from build123d import *

# Parameters (mm, degrees)
F1_DEPTH = 0.75
F2_W     = 0.8
F2_H     = 1
F3_DEPTH = 0.751
F4_W     = 0.8
F4_H     = 1
F5_DEPTH = 0.751
F6_W     = 0.8
F6_H     = 1
F7_DEPTH = 0.751
F8_W     = 0.8
F8_H     = 1
F9_DEPTH = 0.751


with BuildPart() as f1:
    # F0 (on Front) → F1 (new body)
    with BuildSketch(Plane.XZ):
        Polygon((11.8536589885, 0), (-20.1463410115, 0), (-20.1463410115, -3), (-8.1463410115, -3), (-8.1463410115, -1.2), (-0.1463410115, -1.2), (-0.1463410115, -3), (11.8536589885, -3), align=None)
    extrude(amount=F1_DEPTH)

    # F2 (on face) → F3 (cut, through all)
    with BuildSketch(Plane.XZ.offset(0.75)):
        with Locations((-19.2463410115, -0.5)):
            Rectangle(F2_W, F2_H)
    extrude(amount=-F3_DEPTH, mode=Mode.SUBTRACT)

    # F4 (on face) → F5 (cut, through all)
    with BuildSketch(Plane.XZ.offset(0.75)):
        with Locations((-8.5463410115, -0.5)):
            Rectangle(F4_W, F4_H)
    extrude(amount=-F5_DEPTH, mode=Mode.SUBTRACT)

    # F6 (on face) → F7 (cut, through all)
    with BuildSketch(Plane.XZ.offset(0.75)):
        with Locations((0.2536589885, -0.5)):
            Rectangle(F6_W, F6_H)
    extrude(amount=-F7_DEPTH, mode=Mode.SUBTRACT)

    # F8 (on face) → F9 (cut, through all)
    with BuildSketch(Plane.XZ.offset(0.75)):
        with Locations((10.9536589885, -0.5)):
            Rectangle(F8_W, F8_H)
    extrude(amount=-F9_DEPTH, mode=Mode.SUBTRACT)


solid = f1.part
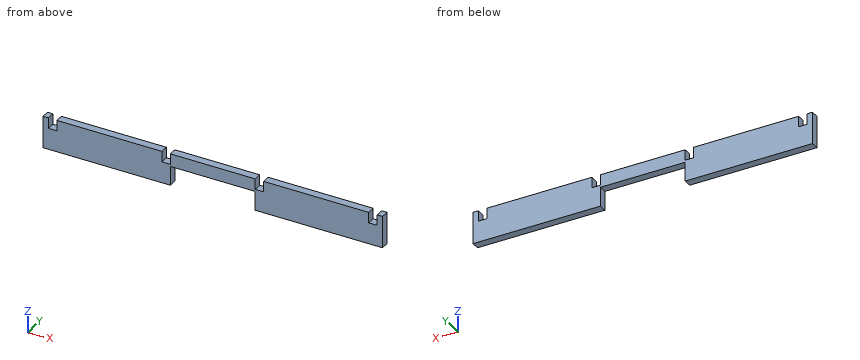
Check sheet for the modelled part. Datum: model origin and axes. Units: mm. Round coordinates to 2 decimals unless told otherwise and drop trailing zeros. Write each loop counter-clockwise with the first axis right and the second up, starting at its lowest first coordinate (ties: lowest second). Pieces come first, ordered by that corner, then holes. Notation, with made-up numbers: (31.25, -28.75) -> (90.25, -28.75) arc R30 ccw to (90.25, 0.25) -> close; hole circle Ø10 at (-7.5, -3.5). An arc over 180 degrees is marked (long way). Answer as CSV lines item,"result". Start each with the question number.
1) Section check A-A on z = -0.7. Enter the section's corners in (x, y).
2) Material ranges on line 1 (X direction, y = -0.05, z = -0.75); line 2 (X direction, y = -0.15, z = -1.35); line 3 (Z direction, x = -2, y = -0.35), recorded low to high. Write a range as from..to.
3) Section check D-D on x = -3.5. Enter the section's corners in (y, z).
4) Section check B-B on z = -2.45. Enter the section's corners in (x, y).
5) Section check C-C on y = -0.35. Enter the section's corners in (x, z).
Found:
1,outline,"(-20.15, -0.75) -> (-19.65, -0.75) -> (-19.65, 0) -> (-20.15, 0) -> close; (-18.85, -0.75) -> (-8.95, -0.75) -> (-8.95, 0) -> (-18.85, 0) -> close; (-8.15, -0.75) -> (-0.15, -0.75) -> (-0.15, 0) -> (-8.15, 0) -> close; (0.65, -0.75) -> (10.55, -0.75) -> (10.55, 0) -> (0.65, 0) -> close; (11.35, -0.75) -> (11.85, -0.75) -> (11.85, 0) -> (11.35, 0) -> close"
2,line 1,"x = -20.15..-19.65, -18.85..-8.95, -8.15..-0.15, 0.65..10.55, 11.35..11.85"
2,line 2,"x = -20.15..-8.15, -0.15..11.85"
2,line 3,"z = -1.2..0"
3,outline,"(-0.75, -1.2) -> (0, -1.2) -> (0, 0) -> (-0.75, 0) -> close"
4,outline,"(-20.15, -0.75) -> (-8.15, -0.75) -> (-8.15, 0) -> (-20.15, 0) -> close; (-0.15, -0.75) -> (11.85, -0.75) -> (11.85, 0) -> (-0.15, 0) -> close"
5,outline,"(-20.15, -3) -> (-8.15, -3) -> (-8.15, -1.2) -> (-0.15, -1.2) -> (-0.15, -3) -> (11.85, -3) -> (11.85, 0) -> (11.35, 0) -> (11.35, -1) -> (10.55, -1) -> (10.55, 0) -> (0.65, 0) -> (0.65, -1) -> (-0.15, -1) -> (-0.15, 0) -> (-8.15, 0) -> (-8.15, -1) -> (-8.95, -1) -> (-8.95, 0) -> (-18.85, 0) -> (-18.85, -1) -> (-19.65, -1) -> (-19.65, 0) -> (-20.15, 0) -> close"
